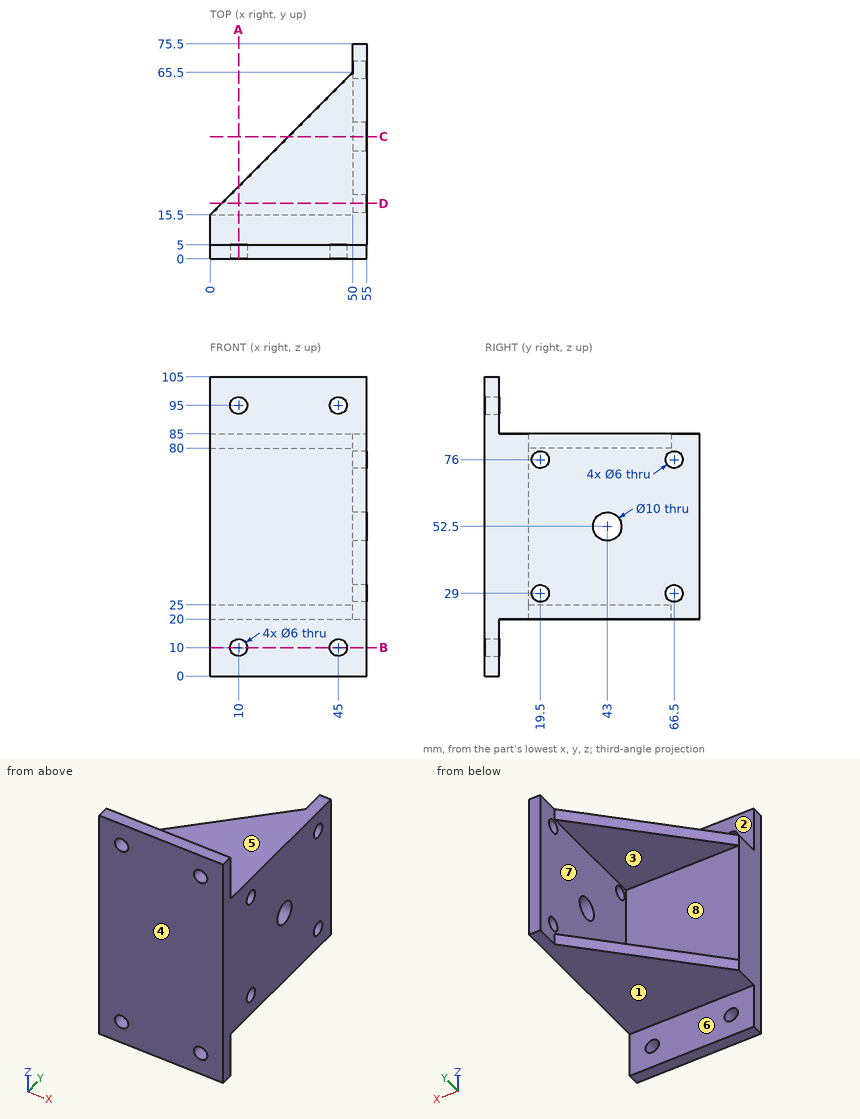
Print and shaded views of the part. All mm, measured from the part's lowest x, y and z. A direction names the side the tool comes from. Round coordinates to 2 decimals unless told otherwise and drop trailing zeros. Write each loop counter-clockwise with the first axis right and the second up, starting at its lowest first coordinate (ties: lowest second). Pieces come first, ordered by that corner, then holes. Notation, with made-up numbers: (-34.75, -9) -> (21.25, -9) arc R14 cw to (21.25, 9) -> close; hole circle Ø4 at (-28, 9.5). An arc over 180 degrees is marked (long way). Return JSON: item names as keys, results as strings. Group by question number.
Q1. Saw through at B-B on z = 10. Write the cut outline in (x, y).
Q2. Saw through at A-A on x = 10. Write the cut outline in (y, z), plus the area to 3 significant figures.
Q3. Pin check, flat tips, straight feed: pin 1 (12 mm diameter, centred on x = 33, z = 23.5, fed in from +Y); pin 2 (5.5 mm diameter, centred on y = 66.5, z = 29, fed in from +X); pin 3 (8 mm diameter, centred on x = 33.5, y = 41.5, fed in from +Z); pin 4 (1.5 mm diameter, centred on x = 29, z = 67, fed in from +Y). Stop position of each tip, or through.
Q4. Saw through at D-D on y = 19.5. Write the cut outline in (x, z), plus the area to 3 significant figures.
Q5. Mould opens along Z. For the marked faces 5, 6, 7 and 8 say: pulls with the +Z half, pulls with the -Z half, needs draft (parallel to the pull), parting line crosses it, or undercut.
Q6. Saw through at C-C on y = 43. Write the cut outline in (x, z).
Q7. Which spindle directions (+Z, -Z, +X, -X, +Y, -Y) get a long thin tool onto all of the face, cutting with end or side? Do the marked faces 1, 2, 3 and 4. Say none if no direction does.
Q8. Probe L1, parallel to Z at x = 45, y = 2.65; L2, parallel to Z at x = 8, y = 17; L3, parallel to X at y = 2, z = 95. List the from-to ranges inside material, lowest first. Write a range as [from, to].
Answer:
{
 "1": {"outline": "(0, 0) -> (7, 0) -> (7, 5) -> (0, 5) -> close; (13, 0) -> (42, 0) -> (42, 5) -> (13, 5) -> close; (48, 0) -> (55, 0) -> (55, 5) -> (48, 5) -> close"},
 "2": {"outline": "(0, 0) -> (5, 0) -> (5, 7) -> (0, 7) -> close; (0, 13) -> (5, 13) -> (5, 20) -> (25.5, 20) -> (25.5, 25) -> (15.5, 25) -> (15.5, 80) -> (25.5, 80) -> (25.5, 85) -> (5, 85) -> (5, 92) -> (0, 92) -> close; (0, 98) -> (5, 98) -> (5, 105) -> (0, 105) -> close", "area": "1,250 mm2"},
 "3": {"pin 1": "y = 54.5", "pin 2": "through", "pin 3": "z = 85", "pin 4": "y = 15.5"},
 "4": {"outline": "(4, 20) -> (55, 20) -> (55, 26) -> (50, 26) -> (50, 25) -> (4, 25) -> close; (4, 80) -> (50, 80) -> (50, 79) -> (55, 79) -> (55, 85) -> (4, 85) -> close; (50, 32) -> (55, 32) -> (55, 73) -> (50, 73) -> close", "area": "725 mm2"},
 "5": {"face 5": "pulls with the +Z half", "face 6": "needs draft", "face 7": "undercut", "face 8": "undercut"},
 "6": {"outline": "(27.5, 20) -> (55, 20) -> (55, 47.5) -> (50, 47.5) -> (50, 25) -> (27.5, 25) -> close; (27.5, 80) -> (50, 80) -> (50, 57.5) -> (55, 57.5) -> (55, 85) -> (27.5, 85) -> close"},
 "7": {"face 1": "-Z, +X, -X, +Y", "face 2": "+Z, +X, -X, +Y", "face 3": "-X, +Y", "face 4": "+Z, -Z, +X, -X, -Y"},
 "8": {"L1": "[0, 7], [13, 92], [98, 105]", "L2": "[20, 25], [80, 85]", "L3": "[0, 7], [13, 42], [48, 55]"}
}
